```python
from build123d import *
from build123d.topology import SkipClean

# Parameters (mm, degrees)
SKETCH1_W           = 2.5
SKETCH1_H           = 2.5
BOSS_EXTRUDE1_DEPTH = 20
CUT_EXTRUDE1_DEPTH  = 21.077973005
CIRPATTERN1_COUNT   = 4
FILLET1_R           = 0.7
SKETCH6_R           = 2.29630994
BOSS_EXTRUDE2_DEPTH = 0.6


with BuildPart() as part:
    # Sketch1 → Boss-Extrude1 (new body)
    with BuildSketch(Plane(origin=(0, 0, 0), x_dir=(1, 0, 0), z_dir=(0, 1, 0))):
        Rectangle(SKETCH1_W, SKETCH1_H)
    extrude(amount=BOSS_EXTRUDE1_DEPTH)

    # Sketch3 → Cut-Extrude1 (cut, symmetric)
    with BuildSketch(Plane(origin=(0, 0, 0), x_dir=(0, 0, -1), z_dir=(1, 0, 0))):
        with BuildLine():
            Line((0, 20), (-2.286909141, 20))
            Line((-2.286909141, 20), (-2.286909141, 0))
            Line((-2.286909141, 0), (-1.031066268, 0))
            Line((-1.031066268, 0), (-1.031066268, 2.793315947))
            ThreePointArc((-1.031066268, 2.793315947), (-1.245689597, 3.603718018), (-0.9, 4.367467579))
            Line((-0.9, 4.367467579), (-0.9, 17.882532421))
            ThreePointArc((-0.9, 17.882532421), (-1.150398729, 19.238960902), (0, 20))
        make_face()
    cut_extrude1 = extrude(amount=CUT_EXTRUDE1_DEPTH, both=True, mode=Mode.SUBTRACT)

    # CirPattern1: Cut-Extrude1 ×4 about axis
    with SkipClean():  # the faces are left unmerged after this step: merging them gives an invalid solid
        cirpattern1_axis = Axis((0, 0, 0), (0, 1, 0))
        for i in range(1, CIRPATTERN1_COUNT):
            add(cut_extrude1.rotate(cirpattern1_axis, i * 360 / CIRPATTERN1_COUNT), mode=Mode.SUBTRACT)

    # Sketch2 → Revolve1 (revolve)
    with BuildSketch(Plane(origin=(0, 0, 0), x_dir=(0, 0, -1), z_dir=(1, 0, 0))):
        with BuildLine():
            Line((2.29630994, 0), (0, 0))
            Line((0, 0), (0, 2.29630994))
            ThreePointArc((0, 2.29630994), (1.623736331, 1.623736331), (2.29630994, 0))
        make_face()
    revolve(axis=Axis((0, 0, 0), (0, 1, 0)))

    # Fillet1
    fillet1_edges = [part.edges().sort_by_distance(p)[0] for p in [
        (0.9, 4.367467579, 0),
        (0, 4.367467579, -0.9),
        (-0.9, 4.367467579, 0),
        (0, 4.367467579, 0.9),
        (0, 17.882532421, -0.9),
        (-0.9, 17.882532421, 0),
        (0, 17.882532421, 0.9),
        (0.9, 17.882532421, 0),
        (-1.031066268, 2.793315947, 0),
        (0, 2.793315947, 1.031066268),
        (1.031066268, 2.793315947, 0),
        (0, 2.793315947, -1.031066268),
        (0.533927601, 1.981126702, -1.031066268),
        (-1.031066268, 2.051814244, 0),
        (0, 2.051814244, 1.031066268),
        (1.031066268, 2.051814244, 0),
    ]]
    fillet(fillet1_edges, radius=FILLET1_R)

    # Sketch6 → Boss-Extrude2 (add)
    with BuildSketch(Plane.XZ):
        with Locations(Location((0, 0, 0), (0, 0, 270))):
            Circle(SKETCH6_R)
    extrude(amount=BOSS_EXTRUDE2_DEPTH)


solid = part.part
```
The listing builds one solid part. Answer for the finished solid, in the listing's coordinates (mm). A direction names the side the tool comes from. Give positions to 0.01 mm unless a question says otherwise; leave off trailing zeros. Order: outer loops, then holes, each group sorted by start corner. A loop starts at its lowest first (then second) coordinate and runs counter-clockwise, first axis right, second up. Notation, with made-up numbers: (30, -18) -> (54, -18) arc R9 cw to (54, -12) -> close; hole circle Ø1 at (88.25, 55). An arc over 180 degrees is marked (long way). Answer as a JSON object with one key per item and string values. Group by question number.
Item 1: Flat-ended cylindrical pins translate along their axes: pin 1 (1.5 mm diameter, centred on y = 16, z = 1.5, fed in from -X); pin 2 (0.5 mm diameter, centred on x = 0, y = 8.5, fed in from +Z); pin 3 (2 mm diameter, centred on y = 12, z = 0, fed in from +X). Find the tip coordinate at first contact, or state that the pin passes through.
Item 2: The part is cut by section B-B on x = -1.6. Write down the section's boundary in (y, z), and give its area (3 significant figures).
Item 3: A tool of negligible diameter and unlimited length cuts with its end or side. For faces 4 (the flat face through (0.9, 11, 0)), 5 (the flat face through (-0.9, 11, 0)), 6 (the flat face through (0, 11, 0.9)), 7 (the flat face through (0, 11, -0.9)), from which of +Z, -Z, +X, -X, +Y, -Y can it reach the whole face along a straight path? Write none if from no direction.
Item 4: Consider L1, parallel to Z at x = 0.35, y = 16.75; L2, parallel to Y at x = -1.6, z = 0. Determine where each line is inside the solid, lowest interval first. Write a range as from..to.
Item 5: The part is cut by section A-A on y = 9.5. Write down the section's boundary in (x, z).
Item 6: Determine the mould class of faces 1 (the flat face through (0, -0.6, 0)), 2 (the cylindrical face through (-1.25, 3.57, 0.02)), 3 (the cylindrical face through (2.277, -0.296, 0.299)) for opening direction Y: pulls with the +Y half, pulls with the -Y half, needs draft (parallel to the pull), parting line crosses it, or undercut.
Result set:
{
 "1": {"pin 1": "x = -0.9", "pin 2": "z = 0.9", "pin 3": "x = 0.9"},
 "2": {"outline": "(-0.6, -1.65) -> (0, -1.65) arc R1.65 ccw to (0, 1.65) -> (-0.6, 1.65) -> close", "area": "6.24 mm²"},
 "3": {"face 4": "+Z, -Z, +X", "face 5": "+Z, -Z, -X", "face 6": "+Z, +X, -X", "face 7": "-Z, +X, -X"},
 "4": {"L1": "-0.9..0.9", "L2": "-0.6..1.65"},
 "5": {"outline": "(-0.9, -0.9) -> (0.9, -0.9) -> (0.9, 0.9) -> (-0.9, 0.9) -> close"},
 "6": {"face 1": "pulls with the -Y half", "face 2": "undercut", "face 3": "needs draft"}
}
